CAD build for the part. Positions are in the model's coordinates, mm. Round coordinates to 2 decimals unless told otherwise and drop trailing zeros. Put each result on its own line as item: value. Start each with the question number.
Item 1: Pin check, flat tip, straight feed: pin 1 Ø3.5 at (x, z) = (4.85, -13.26) entering from -Y (3 decimals). Stop position of the tip, or through.
Item 2: Drill centre line: line 1 (X direction, y = -1.05, z = -12). Where is it in solid material? Low to high. Write a range as from..to.
Item 3: Mould opens along Z. For faces 1 (the flat face through (37, -2, 9.595)), 2 (the flat face through (36, -3.175, -13)), 3 (the cylindrical face through (31.714, -1.565, -12.657)) say: released by +Z, released by -Z, zero draft, split by the parting line, or undercut.
```python
from build123d import *

# Parameters (mm, degrees)
F1_DEPTH = 3.175
F2_DEPTH = 3.175


with BuildPart() as f1:
    # F0 (on Front) → F1 (new body)
    with BuildSketch(Plane.XZ):
        Polygon((-1.5020562172, 9.5954131643), (-1.5020562172, 5.7854131643), (30.2479437828, 5.7854131643), (55.6479437828, 5.7854131643), (74.6979437828, 5.7854131643), (74.6979437828, 9.5954131643), align=None)
        Polygon((74.6979437828, -32.3145868357), (74.6979437828, -36.1245868357), (78.5079437828, -36.1245868357), (78.5079437828, 9.5954131643), (74.6979437828, 9.5954131643), (74.6979437828, 5.7854131643), (74.6979437828, -13.2645868357), align=None)
        Polygon((30.2479437828, -32.3145868357), (-1.5020562172, -32.3145868357), (-1.5020562172, -36.1245868357), (74.6979437828, -36.1245868357), (74.6979437828, -32.3145868357), (55.6479437828, -32.3145868357), align=None)
        Polygon((-1.5020562172, -36.1245868357), (-1.5020562172, -32.3145868357), (-1.5020562172, -13.2645868357), (-1.5020562172, 5.7854131643), (-1.5020562172, 9.5954131643), (-5.3120562172, 9.5954131643), (-5.3120562172, -36.1245868357), align=None)
        with BuildLine():
            ThreePointArc((36.5979437828, -13.2645868357), (38.257752582, -21.0417167691), (42.9479437828, -27.4636184928))
            ThreePointArc((42.9479437828, -27.4636184928), (47.6381349836, -21.0417167691), (49.2979437828, -13.2645868357))
            Line((49.2979437828, -13.2645868357), (36.5979437828, -13.2645868357))
        make_face()
        with BuildLine():
            ThreePointArc((36.5979437828, -13.2645868357), (30.2479437828, -6.9145868357), (23.8979437828, -13.2645868357))
            Line((23.8979437828, -13.2645868357), (28.6604437828, -13.2645868357))
            ThreePointArc((28.6604437828, -13.2645868357), (30.2479437828, -11.6770868357), (31.8354437828, -13.2645868357))
            Line((31.8354437828, -13.2645868357), (36.5979437828, -13.2645868357))
        make_face()
        with BuildLine():
            Line((28.6604437828, -13.2645868357), (23.8979437828, -13.2645868357))
            ThreePointArc((23.8979437828, -13.2645868357), (30.2479437828, -19.6145868357), (36.5979437828, -13.2645868357))
            Line((36.5979437828, -13.2645868357), (31.8354437828, -13.2645868357))
            ThreePointArc((31.8354437828, -13.2645868357), (30.2479437828, -14.8520868357), (28.6604437828, -13.2645868357))
        make_face()
        with BuildLine():
            ThreePointArc((11.1979437828, -13.2645868357), (16.7775596012, -26.7349710173), (30.2479437828, -32.3145868357))
            ThreePointArc((30.2479437828, -32.3145868357), (37.045404593, -31.060570274), (42.9479437828, -27.4636184928))
            ThreePointArc((42.9479437828, -27.4636184928), (38.257752582, -21.0417167691), (36.5979437828, -13.2645868357))
            ThreePointArc((36.5979437828, -13.2645868357), (30.2479437828, -19.6145868357), (23.8979437828, -13.2645868357))
            Line((23.8979437828, -13.2645868357), (11.1979437828, -13.2645868357))
        make_face()
        with BuildLine():
            ThreePointArc((30.2479437828, 5.7854131643), (16.7775596012, 0.2057973459), (11.1979437828, -13.2645868357))
            Line((11.1979437828, -13.2645868357), (23.8979437828, -13.2645868357))
            ThreePointArc((23.8979437828, -13.2645868357), (30.2479437828, -6.9145868357), (36.5979437828, -13.2645868357))
            ThreePointArc((36.5979437828, -13.2645868357), (38.257752582, -5.4874569024), (42.9479437828, 0.9344448214))
            ThreePointArc((42.9479437828, 0.9344448214), (37.045404593, 4.5313966025), (30.2479437828, 5.7854131643))
        make_face()
        with BuildLine():
            Line((36.5979437828, -13.2645868357), (49.2979437828, -13.2645868357))
            ThreePointArc((49.2979437828, -13.2645868357), (47.6381349836, -5.4874569024), (42.9479437828, 0.9344448214))
            ThreePointArc((42.9479437828, 0.9344448214), (38.257752582, -5.4874569024), (36.5979437828, -13.2645868357))
        make_face()
        with BuildLine():
            ThreePointArc((42.9479437828, -27.4636184928), (48.8504829726, -31.060570274), (55.6479437828, -32.3145868357))
            ThreePointArc((55.6479437828, -32.3145868357), (69.1183279644, -26.7349710173), (74.6979437828, -13.2645868357))
            Line((74.6979437828, -13.2645868357), (57.2354437828, -13.2645868357))
            ThreePointArc((57.2354437828, -13.2645868357), (55.6479437828, -14.8520868357), (54.0604437828, -13.2645868357))
            Line((54.0604437828, -13.2645868357), (49.2979437828, -13.2645868357))
            ThreePointArc((49.2979437828, -13.2645868357), (47.6381349836, -21.0417167691), (42.9479437828, -27.4636184928))
        make_face()
        with BuildLine():
            ThreePointArc((42.9479437828, -27.4636184928), (37.045404593, -31.060570274), (30.2479437828, -32.3145868357))
            Line((30.2479437828, -32.3145868357), (55.6479437828, -32.3145868357))
            ThreePointArc((55.6479437828, -32.3145868357), (48.8504829726, -31.060570274), (42.9479437828, -27.4636184928))
        make_face()
    extrude(amount=F1_DEPTH)

    # F0 (on Front) → F2 (join)
    with BuildSketch(Plane.XZ):
        with BuildLine():
            Line((-1.5020562172, 5.7854131643), (-1.5020562172, -13.2645868357))
            ThreePointArc((-1.5020562172, -13.2645868357), (4.8479437828, -6.9145868357), (11.1979437828, -13.2645868357))
            ThreePointArc((11.1979437828, -13.2645868357), (16.7775596012, 0.2057973459), (30.2479437828, 5.7854131643))
            Line((30.2479437828, 5.7854131643), (-1.5020562172, 5.7854131643))
        make_face()
        with BuildLine():
            Line((3.2604437828, -13.2645868357), (-1.5020562172, -13.2645868357))
            ThreePointArc((-1.5020562172, -13.2645868357), (4.8479437828, -19.6145868357), (11.1979437828, -13.2645868357))
            Line((11.1979437828, -13.2645868357), (6.4354437828, -13.2645868357))
            ThreePointArc((6.4354437828, -13.2645868357), (4.8479437828, -14.8520868357), (3.2604437828, -13.2645868357))
        make_face()
        with BuildLine():
            ThreePointArc((11.1979437828, -13.2645868357), (4.8479437828, -6.9145868357), (-1.5020562172, -13.2645868357))
            Line((-1.5020562172, -13.2645868357), (3.2604437828, -13.2645868357))
            ThreePointArc((3.2604437828, -13.2645868357), (4.8479437828, -11.6770868357), (6.4354437828, -13.2645868357))
            Line((6.4354437828, -13.2645868357), (11.1979437828, -13.2645868357))
        make_face()
        with BuildLine():
            Line((-1.5020562172, -13.2645868357), (-1.5020562172, -32.3145868357))
            Line((-1.5020562172, -32.3145868357), (30.2479437828, -32.3145868357))
            ThreePointArc((30.2479437828, -32.3145868357), (16.7775596012, -26.7349710173), (11.1979437828, -13.2645868357))
            ThreePointArc((11.1979437828, -13.2645868357), (4.8479437828, -19.6145868357), (-1.5020562172, -13.2645868357))
        make_face()
        with BuildLine():
            Line((55.6479437828, 5.7854131643), (30.2479437828, 5.7854131643))
            ThreePointArc((30.2479437828, 5.7854131643), (37.045404593, 4.5313966025), (42.9479437828, 0.9344448214))
            ThreePointArc((42.9479437828, 0.9344448214), (48.8504829726, 4.5313966025), (55.6479437828, 5.7854131643))
        make_face()
        with BuildLine():
            Line((57.2354437828, -13.2645868357), (74.6979437828, -13.2645868357))
            ThreePointArc((74.6979437828, -13.2645868357), (69.1183279644, 0.2057973459), (55.6479437828, 5.7854131643))
            ThreePointArc((55.6479437828, 5.7854131643), (48.8504829726, 4.5313966025), (42.9479437828, 0.9344448214))
            ThreePointArc((42.9479437828, 0.9344448214), (47.6381349836, -5.4874569024), (49.2979437828, -13.2645868357))
            Line((49.2979437828, -13.2645868357), (54.0604437828, -13.2645868357))
            ThreePointArc((54.0604437828, -13.2645868357), (55.6479437828, -11.6770868357), (57.2354437828, -13.2645868357))
        make_face()
        with BuildLine():
            ThreePointArc((74.6979437828, -13.2645868357), (69.1183279644, -26.7349710173), (55.6479437828, -32.3145868357))
            Line((55.6479437828, -32.3145868357), (74.6979437828, -32.3145868357))
            Line((74.6979437828, -32.3145868357), (74.6979437828, -13.2645868357))
        make_face()
        with BuildLine():
            ThreePointArc((55.6479437828, 5.7854131643), (69.1183279644, 0.2057973459), (74.6979437828, -13.2645868357))
            Line((74.6979437828, -13.2645868357), (74.6979437828, 5.7854131643))
            Line((74.6979437828, 5.7854131643), (55.6479437828, 5.7854131643))
        make_face()
    extrude(amount=F2_DEPTH)


solid = f1.part
```
Output values:
1. pin 1: y = -3.175
2. line 1: -5.31..3.89, 5.81..29.29, 31.21..54.69, 56.61..78.51
3. face 1: released by +Z
3. face 2: zero draft
3. face 3: undercut
